Autodesk Inventor part; units mm, degrees
ref_plane "YZ Plane" through (0, 0, 0) normal (1, 0, 0) x (0, 1, 0)
ref_plane "XZ Plane" through (0, 0, 0) normal (0, 1, 0) x (-1, 0, 0)
ref_plane "XY Plane" through (0, 0, 0) normal (0, 0, 1) x (1, 0, 0)
sketch "maiin" plane through (0, 0, 0) normal (0, 0, 1) x (1, 0, 0)
  circle A0 centre (-0.0182, -20.0228) radius 2.1844
  circle A1 centre (12.6818, -20.0228) radius 2.1844
  circle A2 centre (-2.8225, 26.9672) radius 2.1844 construction
  arc A3 (-6.3396, -20.5787) -> (-0.0224, -26.3686) centre (-0.0182, -20.0228) ccw
  arc A4 (12.6776, -26.377) -> (18.7159, -18.0313) centre (12.6818, -20.0228) ccw
  arc A5 (3.2076, 28.9574) -> (-8.6291, 29.5373) centre (-2.8225, 26.9672) ccw
  arc A6 (-21.694, 0.0193) -> (-17.0461, -8.7942) centre (-15.8874, -2.5508) ccw
  circle A7 centre (-15.8874, -2.5508) radius 2.0955
  line L0 (18.7159, -18.0313) -> (3.2076, 28.9574)
  line L1 (12.6776, -26.377) -> (-0.0224, -26.3686)
  line L2 (-8.6291, 29.5373) -> (-21.694, 0.0193)
  circle A8 centre (-2.8225, 26.9672) radius 2.1844
  arc A9 (-6.3396, -20.5787) -> (-17.0461, -8.7942) centre (-19.447, -21.7313) ccw
  point P0 (3.1417, -3.9392)
  dimension "d0" = 12.7
  dimension "d1" = 12.7
  dimension "d2" = 4.191
  dimension "d3" = 4.3688
  dimension "d7" = 46.99
sketch "Sketch1" plane through (0, 0, 0) normal (1, 0, 0) x (0, 1, 0)
  circle A0 centre (0.0042, -12.7) radius 2.1844
  circle A1 centre (0, 0) radius 2.1844
  circle A2 centre (-46.9848, -15.5199) radius 2.1844 construction
  arc A3 (0.5622, -19.0212) -> (6.35, -12.7021) centre (0.0042, -12.7) ccw
  arc A4 (6.3542, -0.0021) -> (-1.9935, 6.0334) centre (0, 0) ccw
  arc A5 (-48.977, -9.4905) -> (-49.553, -21.3275) centre (-46.9848, -15.5199) ccw
  arc A6 (-20.0306, -34.3825) -> (-11.2187, -29.7316) centre (-17.4625, -28.575) ccw
  circle A7 centre (-17.4625, -28.575) radius 2.0955
  line L0 (-1.9935, 6.0334) -> (-48.977, -9.4905)
  line L1 (6.3542, -0.0021) -> (6.35, -12.7021)
  line L2 (-49.553, -21.3275) -> (-20.0306, -34.3825)
  circle A8 centre (-46.9848, -15.5199) radius 2.1844
  arc A9 (0.5622, -19.0212) -> (-11.2187, -29.7316) centre (1.7192, -32.1283) ccw
  point P0 (0, 0)
extrude "Extrusion1" add sketch "Sketch1" along normal blind 1.5875
properties part number "bottom_joint_gusset"
The listing builds one solid part. Answer for the finished solid, in the listing's coordinates (mm). Coordinates: 2 decimals unless noted, no trailing zeros. Order: outer loops, then holes, each group sorted by start corner. A loop starts at its lowest first (then second) coordinate and runs counter-clockwise, first axis right, second up. Notation, with made-up numbers: M -36,14 L 7,14 A24 ccw 7,53 Z; hole C 29,-21.5 d11. An arc over 180 degrees is marked long. Answer as a JSON object with one key per item and string values. Group by question number.
1. Straight lines are drawn through the part: line 1 (Y direction, x = 0.6, z = -28.5); line 2 (Z direction, x = 1.3, y = -1.5); line 3 (Z direction, x = 0.1, y = 1). For each, find the intervals that lie inside material, in ascending order.
2. Section A-A on z = -14 is taken. Write down the section's boundary in (x, y), then the cut area to 3 significant figures.
3. Section B-B on y = -18 is taken. Write down the section's boundary in (x, z), then the cut area to 3 significant figures.
4. Section C-C on x = 0.3 is taken. State how many separate pieces and enclosed holes the cut face has, then the cut area to 3 significant figures.
5. Determine the mould class of faces 1 (the cylindrical face through (0.783, -0.469, -10.568)), 2 (the cylindrical face through (0.78, -53.33, -15.32)), 3 (the cylindrical face through (0.783, 4.728, -16.937)) for opening direction Z: released by +Z, released by -Z, zero draft, split by the parting line, or undercut.
6. Section D-D on y = -48 is taken. Write down the section's boundary in (x, z), then the cut area to 3 significant figures.
7. Flat-ended cylindrical pins translate along their axes: P1, Ø5.5, axis at y = -17.46, z = -28.58, coming from the -X side; P2, Ø2.5, axis at y = -46.98, z = -15.52, coming from the -X side. Find the tip coordinate at first contact, or state that the pin passes through.
Values follow:
{
 "1": {"line 1": "-33.33 to -19.56, -15.37 to -10.93", "line 2": "-19.37 to -14.28, -11.12 to -1.59, 1.59 to 6.17", "line 3": "-18.97 to -14.64, -10.76 to -1.94, 1.94 to 6.28"},
 "2": {"outline": "M 0,-53.15 L 1.59,-53.15 L 1.59,-48.55 L 0,-48.55 Z; M 0,-45.42 L 1.59,-45.42 L 1.59,-1.75 L 0,-1.75 Z; M 0,1.76 L 1.59,1.76 L 1.59,6.22 L 0,6.22 Z", "area": "83.7 mm2"},
 "3": {"outline": "M 0,-34.9 L 1.59,-34.9 L 1.59,-30.6 L 0,-30.6 Z; M 0,-26.55 L 1.59,-26.55 L 1.59,0.74 L 0,0.74 Z", "area": "50.2 mm2"},
 "4": {"separate pieces": "1", "enclosed holes": "4", "area": "1,410 mm2"},
 "5": {"face 1": "undercut", "face 2": "split by the parting line", "face 3": "released by -Z"},
 "6": {"outline": "M 0,-22.01 L 1.59,-22.01 L 1.59,-17.45 L 0,-17.45 Z; M 0,-13.59 L 1.59,-13.59 L 1.59,-9.17 L 0,-9.17 Z", "area": "14.3 mm2"},
 "7": {"P1": "x = 0", "P2": "through"}
}
